Can you work these out from the model? Positions are in its coordinate system, mm. A direction names the side the tool comes from. Coordinates: 2 decimals unless noted, no trailing zeros. Order: outer loops, then holes, each group sorted by start corner. A loop starts at its lowest first (then second) coordinate and runs counter-clockwise, first axis right, second up. Notation, with made-up numbers: M 10,7.25 L 53,7.25 A16 ccw 53,36.25 Z; hole C 0.5,-33.75 d1. An arc over 180 degrees is marked long. Answer as a JSON object with one key per item and string values.
Autodesk Inventor part; units mm, degrees
ref_plane "BODY_N_XY" through (107, 0, 0) normal (0, 0, -1) x (1, 0, 0)
ref_plane "BODY_N_YZ" through (107, 0, 0) normal (1, 0, 0) x (0, -1, 0)
ref_plane "BODY_N_ZX" through (107, 0, 0) normal (0, -1, 0) x (0, 0, -1)
sketch "Sketch_8" plane through (0, 0, 0) normal (0, 0, 1) x (1, 0, 0)
  line L0 (0, 0) -> (-8, 0)
  line L1 (-8, 0) -> (-8, 4.3865)
  line L2 (-8, 4.3865) -> (-7.3865, 5)
  line L3 (-7.3865, 5) -> (0, 5)
  line L4 (0, 5) -> (0, 0)
  line L5 (0, 0) -> (-8, 0)
revolve "Revolution1" add sketch "Sketch_8" angle 360 about axis through (0, 0, 0) along (1, 0, 0)
thread "Thread1"
sketch "Sketch_9" plane through (0, 0, 0) normal (1, 0, 0) x (0, 0, -1)
  line L0 (-9.15, 4.0345) -> (-9.15, -4.0345)
  arc A0 (-9.15, -4.0345) -> (-4.0345, -9.15) centre (0, 0) ccw
  line L1 (-4.0345, -9.15) -> (4.0345, -9.15)
  arc A1 (4.0345, -9.15) -> (9.15, -4.0345) centre (0, 0) ccw
  line L2 (9.15, -4.0345) -> (9.15, 4.0345)
  arc A2 (9.15, 4.0345) -> (4.0345, 9.15) centre (0, 0) ccw
  line L3 (4.0345, 9.15) -> (-4.0345, 9.15)
  arc A3 (-4.0345, 9.15) -> (-9.15, 4.0345) centre (0, 0) ccw
extrude "Extrusion1" add sketch "Sketch_9" along normal blind 12.5
sketch "Sketch_11" plane through (12.5, 0, 0) normal (1, 0, 0) x (0, 0, -1)
  circle A0 centre (0, 0) radius 8.7
extrude "Extrusion2" add sketch "Sketch_11" along normal blind 85
sketch "Sketch_10" plane through (97.5, 0, 0) normal (1, 0, 0) x (0, 0, -1)
  line L0 (-9.15, 4.0345) -> (-9.15, -4.0345)
  arc A0 (-9.15, -4.0345) -> (-4.0345, -9.15) centre (0, 0) ccw
  line L1 (-4.0345, -9.15) -> (4.0345, -9.15)
  arc A1 (4.0345, -9.15) -> (9.15, -4.0345) centre (0, 0) ccw
  line L2 (9.15, -4.0345) -> (9.15, 4.0345)
  arc A2 (9.15, 4.0345) -> (4.0345, 9.15) centre (0, 0) ccw
  line L3 (4.0345, 9.15) -> (-4.0345, 9.15)
  arc A3 (-4.0345, 9.15) -> (-9.15, 4.0345) centre (0, 0) ccw
extrude "Extrusion3" add sketch "Sketch_10" along normal blind 9.5
sketch "Sketch7" plane through (0, 0, 0) normal (0, 0, 1) x (1, 0, 0)
  line L0 (8, 9.15) -> (8, 4.15)
  line L1 (8, 2.9566) -> (5.933, 4.15)
  line L2 (5.933, 4.15) -> (5.933, 8.717)
  line L3 (5.933, 8.717) -> (5.5, 9.15)
  line L4 (5.5, 9.15) -> (8, 9.15)
  line L5 (8, 9.15) -> (8, 2.9566)
revolve "Revolution2" cut sketch "Sketch7" angle 360 about axis through (8, 9.15, 0) along (0, 1, 0)
thread "Thread2"
sketch "Sketch_7" plane through (0, 0, 0) normal (0, 0, 1) x (1, 0, 0)
  line L0 (102, 9.15) -> (102, 4.15)
  line L1 (102, 2.9566) -> (99.933, 4.15)
  line L2 (99.933, 4.15) -> (99.933, 8.717)
  line L3 (99.933, 8.717) -> (99.5, 9.15)
  line L4 (99.5, 9.15) -> (102, 9.15)
  line L5 (102, 9.15) -> (102, 2.9566)
revolve "Revolution3" cut sketch "Sketch_7" angle 360 about axis through (102, 9.15, 0) along (0, 1, 0)
thread "Thread3"
sketch "Sketch_16" plane through (0, 0, 0) normal (0, 0, 1) x (1, 0, 0)
  line L0 (77.5, 0) -> (-8, 0)
  line L1 (-8, 0) -> (-8, 2.5)
  line L2 (-8, 2.5) -> (12.5, 2.5)
  line L3 (12.5, 2.5) -> (12.5, 8)
  line L4 (12.5, 8) -> (77.5, 8)
  line L5 (77.5, 8) -> (77.5, 0)
  line L6 (77.5, 0) -> (-8, 0)
revolve "Revolution4" cut sketch "Sketch_16" angle 360 about axis through (77.5, 0, 0) along (1, 0, 0)
ref_plane "BODY_N_XY" through (107, 0, 0) normal (0, 0, -1) x (1, 0, 0)
ref_plane "BODY_N_YZ" through (107, 0, 0) normal (1, 0, 0) x (0, -1, 0)
ref_plane "BODY_N_ZX" through (107, 0, 0) normal (0, -1, 0) x (0, 0, -1)
ref_plane "NUT2_XY" through (107, 0, 0) normal (1, 0, 0) x (0, 0, -1)
ref_plane "NUT2_YZ" through (107, 0, 0) normal (0, 0, -1) x (0, 1, 0)
ref_plane "NUT2_ZX" through (107, 0, 0) normal (0, 1, 0) x (1, 0, 0)
ref_plane "SW1_XY" through (17.5, 0, 0) normal (1, 0, 0) x (0, 0, -1)
ref_plane "SW1_YZ" through (17.5, 0, 0) normal (0, 0, -1) x (0, 1, 0)
ref_plane "SW1_ZX" through (17.5, 0, 0) normal (0, 1, 0) x (1, 0, 0)
ref_plane "SW2_XY" through (92.5, 0, 0) normal (-1, 0, 0) x (0, 0, -1)
ref_plane "SW2_YZ" through (92.5, 0, 0) normal (0, 0, -1) x (0, -1, 0)
ref_plane "SW2_ZX" through (92.5, 0, 0) normal (0, -1, 0) x (-1, 0, 0)
ref_plane "SW_R1_XY" through (17.5, -14.15, 0) normal (1, 0, 0) x (0, 0, -1)
ref_plane "SW_R1_YZ" through (17.5, -14.15, 0) normal (0, 0, -1) x (0, 1, 0)
ref_plane "SW_R1_ZX" through (17.5, -14.15, 0) normal (0, 1, 0) x (1, 0, 0)
ref_plane "SW_R2_XY" through (92.5, -14.15, 0) normal (-1, 0, 0) x (0, 0, -1)
ref_plane "SW_R2_YZ" through (92.5, -14.15, 0) normal (0, 0, -1) x (0, -1, 0)
ref_plane "SW_R2_ZX" through (92.5, -14.15, 0) normal (0, -1, 0) x (-1, 0, 0)
ref_plane "body_XY" through (0, 0, 0) normal (1, 0, 0) x (0, 0, -1)
ref_plane "body_YZ" through (0, 0, 0) normal (0, 0, -1) x (0, 1, 0)
ref_plane "body_ZX" through (0, 0, 0) normal (0, 1, 0) x (1, 0, 0)
properties part number "CJ2B16-60Z(1_0)_BODY" material "ステンレス鋼"
Item 1: I want a section at C-C, the plane y = 6.5. Write out the boundary of the cut face in (x, z).
Answers follow:
{"outline": "M 0,-7.6 L 12.5,-7.6 L 12.5,-5.78 L 97.5,-5.78 L 97.5,-7.6 L 107,-7.6 L 107,7.6 L 97.5,7.6 L 97.5,5.78 L 12.5,5.78 L 12.5,7.6 L 0,7.6 Z; hole C 8,0 d4.13; hole M 12.5,-4.66 L 77.5,-4.66 L 77.5,4.66 L 12.5,4.66 Z; hole C 102,0 d4.13"}
Item 2: I'm going to push flat-ended pins straight in: pin 1 (5 mm diameter, centred on y = -2, z = 5, fed in from -X); pin 2 (1.5 mm diameter, centred on x = 86, z = 3, fed in from +Y); pin 3 (1 mm diameter, centred on x = 83, z = 1, fed in from +Y); pin 4 (6 mm diameter, centred on x = 19, z = -4.5, fed in from +Y). Where does each tip first touch, or does it pass through?
Answers follow:
{"pin 1": "stops at x = -8", "pin 2": "stops at y = 8.4", "pin 3": "stops at y = 8.69", "pin 4": "stops at y = 8.57"}
Item 3: I want a section at D-D, the plane z = -6.5. Write out the boundary of the cut face in (x, y), plus the area to 3 significant figures.
Answers follow:
{"outline": "M 0,-7.6 L 12.5,-7.6 L 12.5,-5.78 L 97.5,-5.78 L 97.5,-7.6 L 107,-7.6 L 107,7.6 L 97.5,7.6 L 97.5,5.78 L 12.5,5.78 L 12.5,7.6 L 0,7.6 Z; hole M 12.5,-4.66 L 77.5,-4.66 L 77.5,4.66 L 12.5,4.66 Z", "area": "711 mm^2"}
Item 4: I want a section at A-A, the plane y = 0. Write out the boundary of the cut face in (x, z).
Answers follow:
{"outline": "M -8,-4.39 L -7.39,-5 L 0,-5 L 0,-9.15 L 12.5,-9.15 L 12.5,-8.7 L 97.5,-8.7 L 97.5,-9.15 L 107,-9.15 L 107,9.15 L 97.5,9.15 L 97.5,8.7 L 12.5,8.7 L 12.5,9.15 L 0,9.15 L 0,5 L -7.39,5 L -8,4.39 L -8,2.5 L 12.5,2.5 L 12.5,8 L 77.5,8 L 77.5,-8 L 12.5,-8 L 12.5,-2.5 L -8,-2.5 Z"}
Item 5: Which directions (+Z, -Z, +X, -X, +Y, -Y) give clear straight access to the entire face, cutting with the end or side of a thin tool? Please do faces 1 (the flat face through (12.5, -2, -2)), 2 (the cylindrical face through (10.065, 6.465, 0.091)), 3 (the flat face through (6, -9.15, 0)), 4 (the cylindrical face through (-3.64, -1.08, -4.88)).
Answers follow:
{"face 1": "none", "face 2": "+Y", "face 3": "+Z, -Z, +X, -X, -Y", "face 4": "-X"}
Item 6: If we mould it in two halves opening along Z, with no side actions, what happens to faces 5 (the cylindrical face through (2.39, -0.54, -2.44)), 6 (the flat face through (102, 0, 9.15)), 7 (the flat face through (102, 9.15, -3))? For each: pulls with the +Z half, pulls with the -Z half, needs draft (parallel to the pull), parting line crosses it, or undercut.
Answers follow:
{"face 5": "undercut", "face 6": "pulls with the +Z half", "face 7": "needs draft"}
Item 7: I want a section at B-B, the plane x = 69.5. Write out the boundary of the cut face in (y, z), plus the area to 3 significant figures.
Answers follow:
{"outline": "C 0,0 d17.4; hole C 0,0 d16", "area": "36.7 mm^2"}
Item 8: Please list where these lines run through material, in increasing order: line 1 (X direction, y = -6, z = 3.25); line 2 (Z direction, x = -2, y = 0); line 3 (X direction, y = 5, z = 7.5).
Answers follow:
{"line 1": "x = 0 to 12.5, 77.5 to 107", "line 2": "z = -5 to -2.5, 2.5 to 5", "line 3": "x = 0 to 12.5, 97.5 to 107"}
